Could you check a few things on this drawing? It's one solid part, dimensions in mm from its lowest x, y, z. Give positions to 0.01 mm unless a question says otherwise; leave off trailing zeros. Loops run counter-clockwise (first coordinate to the right, second up) from the corner with the lowest first, then second, coordinate; pieces in that order, holes last.
1. Imagine slicing it at D-D (z = 3.55). List the corners of the cut face in (x, y) for me (1 decimal), plus the area to 3 significant figures.
2. For P1, Ø2, axis at x = 93.5, z = 0.5, coming from the +Y side (1 decimal), with a flat end and sliding along its axis, tell me the tip position at first contact or that it passes through.
3. I need wall thicknesses on line 1 along X through (y, z) = (26, 4.7) (1 decimal); line 2 along Y through (x, z) = (60, 3.9); line 3 along Y through (x, z) = (59, 5.2). Which ranges of each line are inside material? Lowest first, please.
4. Imagine slicing it at C-C (y = 102.5). List the corners of the cut face in (x, z) for me, plus the area to 3 significant figures.
5. Imagine slicing it at A-A (y = 60). List the corners of the cut face in (x, z) for me.
6. Imagine slicing it at B-B (x = 60). List the corners of the cut face in (y, z) for me.
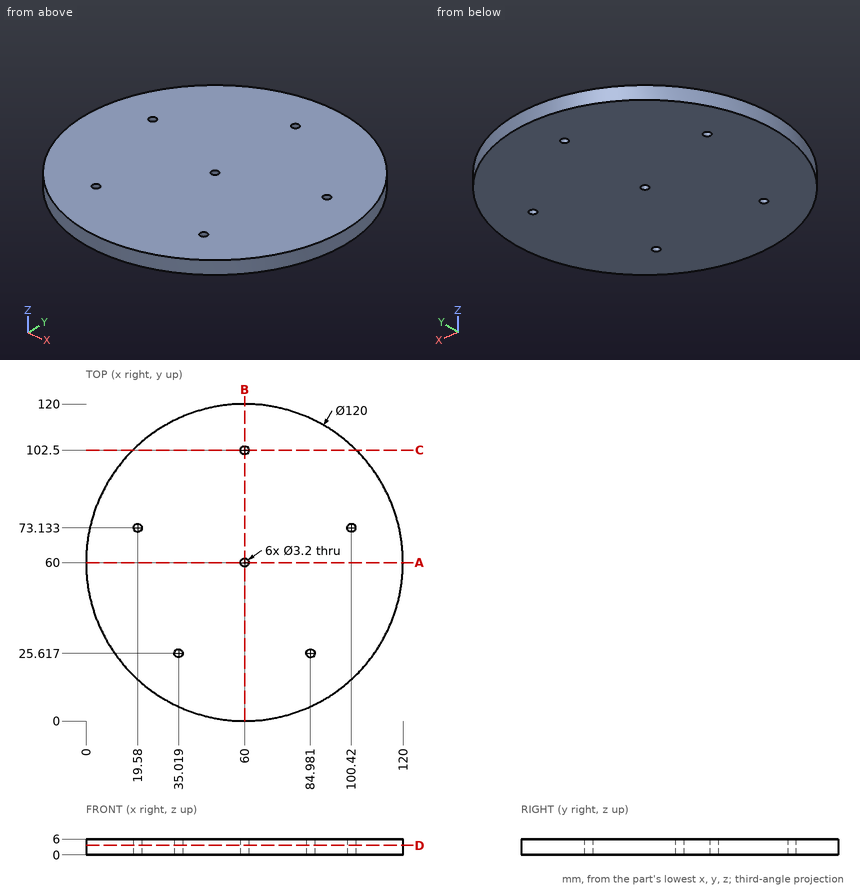
Derived:
1. outline: circle Ø120 at (60, 60); hole circle Ø3.2 at (19.6, 73.1); hole circle Ø3.2 at (35, 25.6); hole circle Ø3.2 at (60, 60); hole circle Ø3.2 at (60, 102.5); hole circle Ø3.2 at (85, 25.6); hole circle Ø3.2 at (100.4, 73.1)
1. area: 11,300 mm2
2. P1: stops at y = 110.4
3. line 1: x = 10.6 to 33.5, 36.6 to 83.4, 86.5 to 109.4
3. line 2: y = 0 to 58.4, 61.6 to 100.9, 104.1 to 120
3. line 3: y = 0.01 to 58.75, 61.25 to 101.25, 103.75 to 119.99
4. outline: (17.65, 0) - (58.4, 0) - (58.4, 6) - (17.65, 6) - close; (61.6, 0) - (102.35, 0) - (102.35, 6) - (61.6, 6) - close
4. area: 489 mm2
5. outline: (0, 0) - (58.4, 0) - (58.4, 6) - (0, 6) - close; (61.6, 0) - (120, 0) - (120, 6) - (61.6, 6) - close
6. outline: (0, 0) - (58.4, 0) - (58.4, 6) - (0, 6) - close; (61.6, 0) - (100.9, 0) - (100.9, 6) - (61.6, 6) - close; (104.1, 0) - (120, 0) - (120, 6) - (104.1, 6) - close
